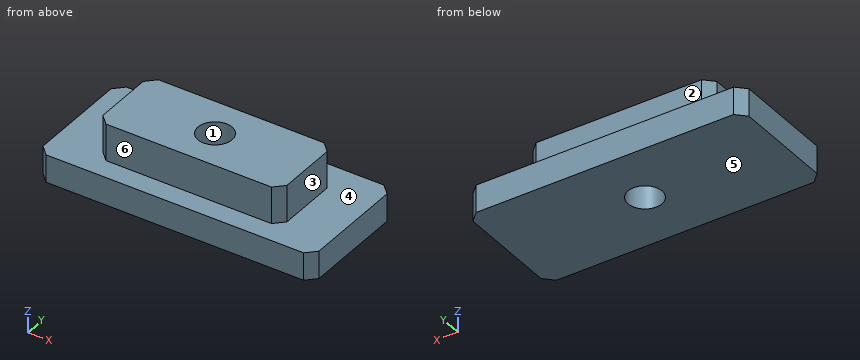
```python
from build123d import *

# Parameters (mm, degrees)
F0_W     = 30
F0_H     = 13
F0_W_2   = 20
F0_H_2   = 8.5
F1_DEPTH = 3
F0_R     = 1.85
F2_DEPTH = 7
F3_SIZE  = 1


with BuildPart() as f1:
    # F0 (on Top) → F1 (new body)
    with BuildSketch(Plane.XY):
        Rectangle(F0_W, F0_H)
        Rectangle(F0_W_2, F0_H_2, mode=Mode.SUBTRACT)
    extrude(amount=F1_DEPTH)

    # F0 (on Top) → F2 (join)
    with BuildSketch(Plane.XY):
        Rectangle(F0_W_2, F0_H_2)
        Circle(F0_R, mode=Mode.SUBTRACT)
    extrude(amount=F2_DEPTH)

    # F3
    f3_edges = [f1.edges().sort_by_distance(p)[0] for p in [
        (-10, -4.25, 5),
        (10, -4.25, 5),
        (10, 4.25, 5),
        (-10, 4.25, 5),
        (-15, 6.5, 1.5),
        (15, 6.5, 1.5),
        (15, -6.5, 1.5),
        (-15, -6.5, 1.5),
    ]]
    chamfer(f3_edges, length=F3_SIZE)


solid = f1.part
```
The model under review builds one solid part; all positions refer to its coordinate system, in mm. Face numbers are marked on the shaded views. A direction names the side the tool comes from. Round coordinates to 2 decimals unless told otherwise and drop trailing zeros. Order: outer loops, then holes, each group sorted by start corner. A loop starts at its lowest first (then second) coordinate and runs counter-clockwise, first axis right, second up. Notation, with made-up numbers: M -9,20.25 L 3,20.25 A6 ccw 3,28.25 Z; hole C -10,69 d6. An arc over 180 degrees is marked long. Use a Markdown table: item, result.
1) Consider section D-D (y = -2.5). Write out the cut boundary in (x, z), then the cut area to 3 significant figures.
Report:
| item | result |
|---|---|
| outline | M -15,0 L 15,0 L 15,3 L 10,3 L 10,7 L -10,7 L -10,3 L -15,3 Z |
| area | 170 mm^2 |
2) Draft analysis for pull direction X (two halves, no side actions). For the marked faces 1, 2 and 3, state which applies: released by +X, released by -X, zero draft, split by the parting line, or undercut.
Report:
| item | result |
|---|---|
| face 1 | undercut |
| face 2 | zero draft |
| face 3 | released by +X |
3) Tool access review of the marked faces 4, 5 and 6: name each direction out of +Z, -Z, +X, -X, +Y, -Y from which nothing blocks a thin tool from reaching the whole face with its end or side.
Report:
| item | result |
|---|---|
| face 4 | +Z |
| face 5 | -Z, +X, -X, +Y, -Y |
| face 6 | +Z, +X, -X, -Y |
4) Insertion check: pin 1 (1.2 mm diameter, centred on y = -0.5, z = 4.5, fed in from +X); pin 2 (2 mm diameter, centred on x = 1.5, z = 5.5, fed in from +Y); pin 3 (3 mm diameter, centred on y = -1.5, z = 5, fed in from -X); pin 4 (2 mm diameter, centred on x = 0, y = 0, fed in from -Z). Each pin has a flat end and moves straight along its axis. Give the tip position at first contact, or say it passes through.
Report:
| item | result |
|---|---|
| pin 1 | x = 10 |
| pin 2 | y = 4.25 |
| pin 3 | x = -10 |
| pin 4 | through |
5) Consider section C-C (z = 3.75). Write out the cut boundary in (x, y).
Report:
| item | result |
|---|---|
| outline | M -10,-3.25 L -9,-4.25 L 9,-4.25 L 10,-3.25 L 10,3.25 L 9,4.25 L -9,4.25 L -10,3.25 Z; hole C 0,0 d3.7 |
6) Consider section A-A (y = 0). Write out the cut boundary in (x, z), then the cut area to 3 significant figures.
Report:
| item | result |
|---|---|
| outline | M -15,0 L -1.85,0 L -1.85,7 L -10,7 L -10,3 L -15,3 Z; M 1.85,0 L 15,0 L 15,3 L 10,3 L 10,7 L 1.85,7 Z |
| area | 144 mm^2 |
7) Wall thickness on line 1 along Y through (x, z) = (0, 4.25); line 2 along Y through (x, z) = (0, 2.25); line 3 along X through (y, z) = (-0.5, 1.75): over which ranges is each line inside the solid? List them lowest first. Write a range as [from, to].
Report:
| item | result |
|---|---|
| line 1 | [-4.25, -1.85], [1.85, 4.25] |
| line 2 | [-6.5, -1.85], [1.85, 6.5] |
| line 3 | [-15, -1.78], [1.78, 15] |
8) Consider section B-B (x = 0). Write out the cut boundary in (y, z).
Report:
| item | result |
|---|---|
| outline | M -6.5,0 L -1.85,0 L -1.85,7 L -4.25,7 L -4.25,3 L -6.5,3 Z; M 1.85,0 L 6.5,0 L 6.5,3 L 4.25,3 L 4.25,7 L 1.85,7 Z |
